Geometry check sheet. Reference: the model listing, model coordinates, mm. Round coordinates to 2 decimals unless told otherwise and drop trailing zeros. Write each loop counter-clockwise with the first axis right and the second up, starting at its lowest first coordinate (ties: lowest second). Pieces come first, ordered by that corner, then holes. Notation, with made-up numbers: (22, -19.75) -> (33, -19.75) arc R22 ccw to (33, 11.25) -> close; hole circle Ø1 at (-21, 74). An arc over 180 degrees is marked (long way). Use a Markdown table: item, result.
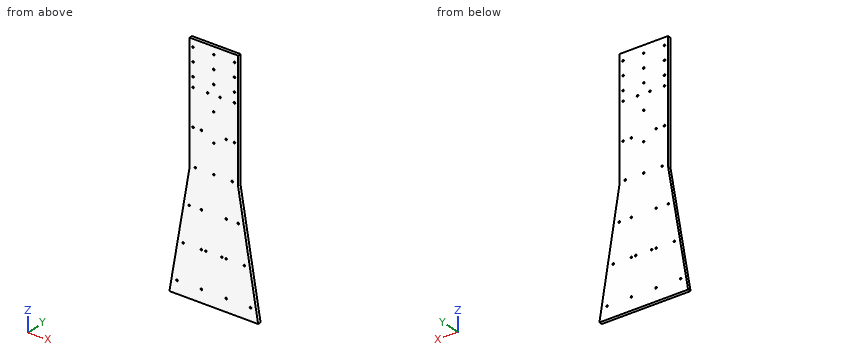
Autodesk Inventor part; units mm, degrees
ref_plane "YZ Plane" through (0, 0, 0) normal (1, 0, 0) x (0, 1, 0)
ref_plane "XZ Plane" through (0, 0, 0) normal (0, 1, 0) x (-1, 0, 0)
ref_plane "XY Plane" through (0, 0, 0) normal (0, 0, 1) x (1, 0, 0)
sketch "Эскиз1" plane through (0, 0, 0) normal (0, 1, 0) x (-1, 0, 0)
  line L0 (0, 0) -> (0, 458.3537) construction
  line L1 (0, 0) -> (0, -395.9132) construction
  line L2 (0, 0) -> (0, -1420) construction
  line L3 (0, -1420) -> (-240, -1420) construction
  line L4 (0, -1420) -> (240, -1420) construction
  line L5 (-240, -1420) -> (-11.5109, -68.1064) construction
  line L6 (-45, 13.7558) -> (45, 13.7558)
  line L7 (45, 13.7558) -> (45, -206.2442)
  line L8 (45, -206.2442) -> (-45, -206.2442) construction
  line L9 (-45, -206.2442) -> (-45, 13.7558)
  line L10 (-45, 13.7558) -> (45, -206.2442) construction
  line L11 (45, 13.7558) -> (-45, -206.2442) construction
  line L12 (-251.832, -1430) -> (-82.1831, -426.2442) construction
  line L13 (-45, -206.2442) -> (45, -206.2442) construction
  line L14 (45, -206.2442) -> (45, -426.2442) construction
  line L15 (45, -426.2442) -> (-45, -426.2442) construction
  line L16 (-45, -426.2442) -> (-45, -206.2442) construction
  line L17 (0, -426.2442) -> (-82.1831, -426.2442)
  line L18 (-82.1831, -426.2442) -> (-45, -206.2442)
  line L19 (0, -426.2442) -> (82.1831, -426.2442)
  line L20 (82.1831, -426.2442) -> (45, -206.2442)
  circle A0 centre (-11.5109, -68.1064) radius 1.5
  line L21 (-11.5109, -68.1064) -> (0, 0) construction
  circle A1 centre (-22.8432, -135.1555) radius 1.5
  circle A2 centre (-34.1754, -202.2045) radius 1.5
  circle A3 centre (-45.5077, -269.2536) radius 1.5
  circle A4 centre (-56.8399, -336.3027) radius 1.5
  circle A5 centre (-68.1721, -403.3518) radius 1.5
  circle A6 centre (11.5109, -68.1064) radius 1.5
  circle A7 centre (22.8432, -135.1555) radius 1.5
  circle A8 centre (34.1754, -202.2045) radius 1.5
  circle A9 centre (45.5077, -269.2536) radius 1.5
  circle A10 centre (56.8399, -336.3027) radius 1.5
  circle A11 centre (68.1721, -403.3518) radius 1.5
  line L22 (0, -96.2442) -> (0, -202.2045)
  circle A12 centre (0, -202.2045) radius 1.5
  circle A13 centre (0, -149.2045) radius 1.5
  circle A14 centre (0, -96.2045) radius 1.5
  point P0 (0, -96.2442)
  dimension "d16" = 240
  dimension "d17" = 180
  dimension "d18" = 1420
  dimension "d21" = 90
  dimension "d22" = 220
  dimension "d24" = 10
  dimension "d25" = 90
  dimension "d26" = 220
  dimension "d27" = 3
  dimension "d30" = 68
  dimension "d39" = 53
extrude "Выдавливание1" add sketch "Эскиз1" along normal blind 6 contours L6 L7 L20 L19 L17 L18 L9 | A12 | A13 L22 | L22 A13 | A14
extrude "Выдавливание2" cut sketch "Эскиз1" along normal blind 10 contours A12 | A13 L22 | L22 A13 | A14
sketch "Эскиз2" plane through (0, 6, 0) normal (0, 1, 0) x (1, 0, 0)
  circle A0 centre (-45.5077, 269.2536) radius 1.5
  circle A1 centre (-56.8399, 336.3027) radius 1.5
  circle A2 centre (0, 202.2045) radius 1.5
  circle A3 centre (0, 149.2045) radius 1.5
  circle A4 centre (0, 96.2045) radius 1.5
  line L0 (45, 206.2442) -> (82.1831, 426.2442)
  line L1 (82.1831, 426.2442) -> (-82.1831, 426.2442)
  line L2 (-82.1831, 426.2442) -> (-45, 206.2442)
  line L3 (-45, 206.2442) -> (-45, -13.7558)
  line L4 (-45, -13.7558) -> (45, -13.7558)
  line L5 (45, -13.7558) -> (45, 206.2442)
  circle A5 centre (11.5109, 68.1064) radius 1.5
  circle A6 centre (22.8432, 135.1555) radius 1.5
  circle A7 centre (34.1754, 202.2045) radius 1.5
  circle A8 centre (-11.5109, 68.1064) radius 1.5
  circle A9 centre (-22.8432, 135.1555) radius 1.5
  circle A10 centre (-34.1754, 202.2045) radius 1.5
  circle A11 centre (45.5077, 269.2536) radius 1.5
  circle A12 centre (56.8399, 336.3027) radius 1.5
  circle A13 centre (68.1721, 403.3518) radius 1.5
  circle A14 centre (-45.5077, 269.2536) radius 1.5
  circle A15 centre (-56.8399, 336.3027) radius 1.5
  circle A16 centre (-68.1721, 403.3518) radius 1.5
  line L6 (-82.1831, 426.2442) -> (-45, 206.2442)
  line L7 (-55.6495, 269.2536) -> (55.6495, 269.2536)
  line L8 (45, 206.2442) -> (82.1831, 426.2442)
  line L9 (-66.9817, 336.3027) -> (66.9817, 336.3027)
  line L10 (-78.314, 403.3518) -> (78.314, 403.3518)
  circle A17 centre (-22.8432, 269.2536) radius 1.5
  circle A18 centre (22.8432, 269.2536) radius 1.5
  circle A19 centre (-22.8432, 336.3027) radius 1.5
  circle A20 centre (22.8432, 336.3027) radius 1.5
  circle A21 centre (-22.8432, 403.3518) radius 1.5
  circle A22 centre (22.8432, 403.3518) radius 1.5
  point P0 (0, 0)
extrude "Выдавливание3" cut sketch "Эскиз2" against normal blind 10 contours A17 L7 | L7 A17 | A18 L7 | L7 A18 | A19 L9 | L9 A19 | A21 L10 | L10 A21 | A20 L9 | L9 A20 | A22 L10 | L10 A22
sketch "Эскиз3" plane through (0, 6, 0) normal (0, 1, 0) x (1, 0, 0)
  circle A0 centre (-22.8432, 336.3027) radius 1.5
  circle A1 centre (22.8432, 403.3518) radius 1.5
  circle A2 centre (22.8432, 269.2536) radius 1.5
  circle A3 centre (22.8432, 336.3027) radius 1.5
  circle A4 centre (-22.8432, 403.3518) radius 1.5
  circle A5 centre (-22.8432, 269.2536) radius 1.5
  circle A6 centre (0, 202.2045) radius 1.5
  circle A7 centre (0, 149.2045) radius 1.5
  circle A8 centre (0, 96.2045) radius 1.5
  line L0 (45, 206.2442) -> (82.1831, 426.2442)
  line L1 (82.1831, 426.2442) -> (-82.1831, 426.2442)
  line L2 (-82.1831, 426.2442) -> (-45, 206.2442)
  line L3 (-45, 206.2442) -> (-45, -13.7558)
  line L4 (-45, -13.7558) -> (45, -13.7558)
  line L5 (45, -13.7558) -> (45, 206.2442)
  circle A9 centre (11.5109, 68.1064) radius 1.5
  circle A10 centre (22.8432, 135.1555) radius 1.5
  circle A11 centre (34.1754, 202.2045) radius 1.5
  circle A12 centre (-11.5109, 68.1064) radius 1.5
  circle A13 centre (-22.8432, 135.1555) radius 1.5
  circle A14 centre (-34.1754, 202.2045) radius 1.5
  circle A15 centre (45.5077, 269.2536) radius 1.5
  circle A16 centre (56.8399, 336.3027) radius 1.5
  circle A17 centre (68.1721, 403.3518) radius 1.5
  circle A18 centre (-45.5077, 269.2536) radius 1.5
  circle A19 centre (-56.8399, 336.3027) radius 1.5
  circle A20 centre (-68.1721, 403.3518) radius 1.5
  line L6 (-45, 206.2442) -> (-45, -13.7558)
  line L7 (-45, 68.1064) -> (45, 68.1064)
  line L8 (45, -13.7558) -> (45, 206.2442)
  line L9 (-45, 135.1555) -> (45, 135.1555)
  circle A21 centre (-38.4, 135.1555) radius 1.5
  circle A22 centre (-38.4, 68.1064) radius 1.5
  circle A23 centre (38.4, 68.1064) radius 1.5
  circle A24 centre (38.4, 135.1555) radius 1.5
  line L10 (-39.9, 0) -> (38.4, 0)
  line L11 (0, 0) -> (0, 68.1064)
  circle A25 centre (38.4, 0) radius 1.5
  circle A26 centre (0, 0) radius 1.5
  circle A27 centre (-38.4, 0) radius 1.5
  line L12 (-39.9, 25) -> (38.4, 25)
  circle A28 centre (-38.4, 25) radius 1.5
  circle A29 centre (0, 25) radius 1.5
  circle A30 centre (38.4, 25) radius 1.5
  line L13 (-39.9, 50) -> (38.4, 50)
  circle A31 centre (-38.4, 50) radius 1.5
  circle A32 centre (0, 50) radius 1.5
  circle A33 centre (38.4, 50) radius 1.5
  dimension "d48" = 3
  dimension "d49" = 6.6
  dimension "d50" = 6.6
  dimension "d51" = 6.6
  dimension "d52" = 6.6
  dimension "d62" = 25
extrude "Выдавливание4" cut sketch "Эскиз3" against normal blind 10 contours A33 | A30 | A25 | A27 L10 | L10 A27 | A26 L10 L11 | L11 L10 A26 | A28 L12 | L12 A28 | A29 L12 L11 | L11 L12 A29 | A31 L13 | L13 A31 | A32 L13 L11 | L11 L13 A32 | A24 L9 | L9 A24 | A23 L7 | L7 A23 | A21 L9 | L9 A21 | A22 L7 | L7 A22 | L13 A32 L11 | L11 A32 L13 | L12 A29 L11 | L11 A29 L12 | L10 A26
sketch "Эскиз4" plane through (0, 0, 0) normal (0, -1, 0) x (1, 0, 0)
  circle A0 centre (-22.8432, -336.3027) radius 1.5
  circle A1 centre (22.8432, -336.3027) radius 1.5
  circle A2 centre (-22.8432, -336.3027) radius 1.5
  line L0 (-22.8432, -336.3027) -> (22.8432, -336.3027)
  line L1 (0, -336.3027) -> (14.75, -336.3027)
  line L2 (0, -336.3027) -> (-14.75, -336.3027)
  circle A3 centre (-14.75, -336.3027) radius 1.45
  circle A4 centre (14.75, -336.3027) radius 1.45
  point P0 (0, 0)
  dimension "d69" = 14.75
  dimension "d70" = 14.75
  dimension "d71" = 2.9
  dimension "d72" = 2.9
extrude "Выдавливание5" cut sketch "Эскиз4" against normal through all contours A4 L0 | L0 A4 | A3 L0 | L0 A3
properties part number "шея2,0"
(1) Section check C-C on z = -238.5. Record the cut outline in (x, y), plus the area to 3 significant figures.
A:
| item | result |
|---|---|
| outline | (-50.45, 0) -> (50.45, 0) -> (50.45, 6) -> (-50.45, 6) -> close |
| area | 605 mm2 |
(2) Thickness scan on line 1 (Z direction, x = 38.4, y = 1.8); line 2 (X direction, y = 2.95, z = -50); line 3 (Z direction, x = 34, y = 2.65). Record the ranges inside material, lowest first.
A:
| item | result |
|---|---|
| line 1 | z = -426.24 to -136.66, -133.66 to -69.61, -66.61 to -51.5, -48.5 to -26.5, -23.5 to -1.5, 1.5 to 13.76 |
| line 2 | x = -45 to -39.9, -36.9 to -1.5, 1.5 to 36.9, 39.9 to 45 |
| line 3 | z = -426.24 to -203.69, -200.71 to 13.76 |
(3) Section check A-A on z = -120. Record the cut outline in (x, y), plus the area to 3 significant figures.
A:
| item | result |
|---|---|
| outline | (-45, 0) -> (45, 0) -> (45, 6) -> (-45, 6) -> close |
| area | 540 mm2 |
(4) Gauge pin test, flat ends, axial feed: pin 1 Ø2.5 at (x, z) = (-56.84, -336.3) entering from +Y; pin 2 Ø1 at (y, z) = (2.5, -280) entering from -X. Record the tip position at first contact, or that the pin passes through.
A:
| item | result |
|---|---|
| pin 1 | passes through |
| pin 2 | stops at x = -57.55 |
(5) Section check B-B on y = 1.15. State how many separate pieces and enclosed holes the cut face has, plus the area to 3 significant figures.
A:
| item | result |
|---|---|
| separate pieces | 1 |
| enclosed holes | 36 |
| area | 47,500 mm2 |
